from build123d import *

# Parameters (mm, degrees)
F2_W     = 62.104048
F2_H     = 22.225
F3_DEPTH = 12.7


with BuildPart() as f1:
    # F0 (on Front) → F1 (revolve)
    with BuildSketch(Plane.XZ):
        with BuildLine():
            Line((0, 22.225), (0, -22.225))
            ThreePointArc((0, -22.225), (22.225, 0), (0, 22.225))
        make_face()
    revolve(axis=Axis((0, 0, 0), (0, 0, -1)))

    # F2 (on Front) → F3 (join, symmetric)
    with BuildSketch(Plane.XZ):
        with Locations((-1.405022, 11.1125)):
            Rectangle(F2_W, F2_H)
    extrude(amount=F3_DEPTH, both=True)


solid = f1.part
Check sheet for the modelled part. Datum: model origin and axes. Units: mm. A direction names the side the tool comes from. Coordinates: 2 decimals unless noted, no trailing zeros. Write each loop counter-clockwise with the first axis right and the second up, starting at its lowest first coordinate (ties: lowest second). Pieces come first, ordered by that corner, then holes. Notation, with made-up numbers: M 85,13.25 L 143,13.25 A17 cw 143,21.25 Z; hole C 53.5,-23 d5. An arc over 180 degrees is marked long. Answer as CSV lines item,"result".
Q1. Go/stop test with flat-tipped pins: pin 1 (2 mm diameter, centred on x = -15.5, y = -0.5, fed in from -Z); pin 2 (18 mm diameter, centred on x = -4, z = 14, fed in from +Y); pin 3 (6 mm diameter, centred on y = -6, z = -16, fed in from -X); pin 4 (8 mm diameter, centred on x = -25.5, z = -7, fed in from -Y). Record where each tip stops, or that it passes through.
Check result:
pin 1,"z = -16.84"
pin 2,"y = 21.52"
pin 3,"x = -17.19"
pin 4,"through"
Q2. Cross-section at D-D (y = -3.5). Record the boundary of the cut face in (x, z) (3 decimals).
Check result:
outline,"M -32.457,0 L -21.948,0 A21.948 ccw 21.948,0 L 29.647,0 L 29.647,22.225 L -32.457,22.225 Z"
Q3. Material ranges on probe 1 along Y at (x, z) = (22.5, 19.5); probe 2 along Z at (x, y) = (-5.5, 8.5) (3 decimals); probe 3 along Z at (x, y) = (6, 10) (3 decimals), recorded low to high. Write a range as from..to.
Check result:
probe 1,"-12.7..12.7"
probe 2,"-19.785..22.225"
probe 3,"-18.92..22.225"
Q4. Cross-section at B-B (y = 6). Record the boundary of the cut face in (x, z) (3 decimals), then the cut area to 3 significant figures.
Check result:
outline,"M -32.457,0 L -21.4,0 A21.4 ccw 21.4,0 L 29.647,0 L 29.647,22.225 L -32.457,22.225 Z"
area,"2,100 mm^2"
Q5. Set-up check for faces 1 (the face through (-2, -12.7, 19)), 2 (the face through (-32.457, 0, 11)), 3 (the face through (-2, 12.7, 19)): record each of +Z, -Z, +X, -X, +Y, -Y from which the full face is reachable in a straight line by a thin tool's end or side.
Check result:
face 1,"+Z, -Y"
face 2,"+Z, -Z, -X, +Y, -Y"
face 3,"+Z, +Y"
Q6. Cross-section at A-A (z = 12.5). Record the boundary of the cut face in (x, y), then the cut area to 3 significant figures.
Check result:
outline,"M -32.46,-12.7 L -13.28,-12.7 A18.38 ccw 13.28,-12.7 L 29.65,-12.7 L 29.65,12.7 L 13.28,12.7 A18.38 ccw -13.28,12.7 L -32.46,12.7 Z"
area,"1,790 mm^2"
Q7. Cross-section at C-C (x = -23). Record the boundary of the cut face in (y, z) (3 decimals), then the cut area to 3 significant figures.
Check result:
outline,"M -12.7,0 L 12.7,0 L 12.7,22.225 L -12.7,22.225 Z"
area,"565 mm^2"
